```python
from build123d import *

# Parameters (mm, degrees)
EXTRUDE_5_DEPTH     = 19
SKETCH_6_R          = 4.25
CUT_EXTRUDE_1_DEPTH = 19


with BuildPart() as part:
    # 草图5 → 凸台-拉伸5 (new body)
    with BuildSketch(Plane(origin=(0, 0, 0), x_dir=(0, 0, -1), z_dir=(1, 0, 0))):
        Polygon((12.1, 0), (-12.1, 0), (-12.1, -7.1), (-32, -7.1), (-32, -8.9), (-10.3, -8.9), (-10.3, -1.8), (10.3, -1.8), (10.3, -8.9), (32, -8.9), (32, -7.1), (12.1, -7.1), align=None)
    extrude(amount=EXTRUDE_5_DEPTH)

    # 草图6 → 切除-拉伸1 (cut)
    with BuildSketch(Plane(origin=(0, -7.1, 0), x_dir=(1, 0, 0), z_dir=(0, 1, 0))):
        with Locations(Location((9.5, -22.6, 0), (0, 0, 270))):
            Circle(SKETCH_6_R)
        with Locations(Location((9.5, 22.6, 0), (0, 0, 270))):
            Circle(SKETCH_6_R)
    extrude(amount=-CUT_EXTRUDE_1_DEPTH, mode=Mode.SUBTRACT)


solid = part.part
```
The model under review builds one solid part; all positions refer to its coordinate system, in mm. A direction names the side the tool comes from. Round coordinates to 2 decimals unless told otherwise and drop trailing zeros. Write each loop counter-clockwise with the first axis right and the second up, starting at its lowest first coordinate (ties: lowest second). Pieces come first, ordered by that corner, then holes. Notation, with made-up numbers: (34.5, -8) - (68.5, -8) arc R23 cw to (68.5, 12) - close; hole circle Ø6 at (-14, 13). An arc over 180 degrees is marked (long way). Answer as CSV lines item,"result". Start each with the question number.
(1) For faces 4 (the flat face through (9, -5, -10.3)), 5 (the flat face through (5, -8.9, 21)), 6 (the flat face through (5, -7.1, 22)), 7 (the flat face through (9, -8, -32)), 8 (the flat face through (5, -7.1, -22)), list the 3-axis set-ups (+Z, -Z, +X, -X, +Y, -Y) from which the entire face can be reached by the end or side of a thin tool; tool diameter is ignored.
(2) We need section A-A on z = 22.6. State the section outline as (x, y) points, plus the area to 3 significant figures.
(3) To check wall thickness, follow line 1 (X direction, y = -7.8, z = 22.6); line 2 (Z direction, x = 8, y = -6.5); line 3 (Z direction, x = 11, y = -7.75). State the ranges of each line that lie inside material, in increasing order.
(4) We need section C-C on x = 9.5. State the section outline as (y, z) points, plus the area to 3 significant figures.
(5) For pin 1 Ø3 at (y, z) = (-3.5, -8.5) entering from +X; pin 2 Ø3 at (x, y) = (5, -1) entering from +Z; pin 3 Ø9.5 at (x, z) = (12, -1) entering from -Y; pin 4 Ø2 at (x, z) = (13.5, -16) entering from +Y, all flat-tipped, find the tip position at first contact; note any pin that passes through.
(6) Draft analysis for pull direction X (two halves, no side actions). For faces 1 (the flat face through (9, -4, 12.1)), 2 (the flat face through (0, -1, 0)), 3 (the cylindrical face through (6.91, -7.99, -25.97)), state which applies: pulls with the +X half, pulls with the -X half, needs draft (parallel to the pull), parting line crosses it, or undercut.
(7) We need section B-B on y = -2.5. State the section outline as (x, z) points.
(8) We need section D-D on x = 15.75. State the section outline as (y, z) points, plus the area to 3 significant figures.
Worked answers:
1,face 4,"+X, -X, -Y"
1,face 5,"+Z, -Z, +X, -X, -Y"
1,face 6,"+Z, +X, -X, +Y"
1,face 7,"-Z, +X, -X, +Y, -Y"
1,face 8,"-Z, +X, -X, +Y"
2,outline,"(0, -8.9) - (5.25, -8.9) - (5.25, -7.1) - (0, -7.1) - close; (13.75, -8.9) - (19, -8.9) - (19, -7.1) - (13.75, -7.1) - close"
2,area,"18.9 mm²"
3,line 1,"0 to 5.25, 13.75 to 19"
3,line 2,"-12.1 to -10.3, 10.3 to 12.1"
3,line 3,"-32 to -26.58, -18.62 to -10.3, 10.3 to 18.62, 26.58 to 32"
4,outline,"(-8.9, -32) - (-7.1, -32) - (-7.1, -26.85) - (-8.9, -26.85) - close; (-8.9, -18.35) - (-7.1, -18.35) - (-7.1, -12.1) - (0, -12.1) - (0, 12.1) - (-7.1, 12.1) - (-7.1, 18.35) - (-8.9, 18.35) - (-8.9, 10.3) - (-1.8, 10.3) - (-1.8, -10.3) - (-8.9, -10.3) - close; (-8.9, 26.85) - (-7.1, 26.85) - (-7.1, 32) - (-8.9, 32) - close"
4,area,"110 mm²"
5,pin 1,"through"
5,pin 2,"z = 12.1"
5,pin 3,"y = -1.8"
5,pin 4,"y = -7.1"
6,face 1,"needs draft"
6,face 2,"pulls with the -X half"
6,face 3,"undercut"
7,outline,"(0, -12.1) - (19, -12.1) - (19, -10.3) - (0, -10.3) - close; (0, 10.3) - (19, 10.3) - (19, 12.1) - (0, 12.1) - close"
8,outline,"(-8.9, -32) - (-7.1, -32) - (-7.1, -12.1) - (0, -12.1) - (0, 12.1) - (-7.1, 12.1) - (-7.1, 32) - (-8.9, 32) - (-8.9, 10.3) - (-1.8, 10.3) - (-1.8, -10.3) - (-8.9, -10.3) - close"
8,area,"141 mm²"
